Check sheet for the drawn part. Datum: minimum x, y, z corner. Units: mm. A direction names the side the tool comes from. Coordinates: 2 decimals unless noted, no trailing zeros. Order: outer loops, then holes, each group sorted by start corner. A loop starts at its lowest first (then second) coordinate and runs counter-clockwise, first axis right, second up. Notation, with made-up numbers: M 49.25,-23.75 L 75.25,-23.75 A26 cw 75.25,-3.75 Z; hole C 31.25,-30 d1. An arc over 180 degrees is marked long. Return JSON: item names as keys, results as strings. Group by question number.
Q1. Section check B-B, the plane z = 14.5. Enter the section's corners in (x, y) (1 decimal).
Q2. Mould release check, pull along Z, two halves, no side actions. Record for the marked faces 1, 2, 3 and 4: pulls with the +Z half, pulls with the -Z half, needs draft (parallel to the pull), parting line crosses it, or undercut.
Q3. Go/stop test with flat-tipped pins: pin 1 Ø14 at (x, z) = (15, 13.5) entering from -Y; pin 2 Ø0.9 at (x, y) = (11.5, 1) entering from +Z; pin 3 Ø5.5 at (x, z) = (12.5, 12.5) entering from +Y. Record where each tip stops, or that it passes through.
Q4. Thickness scan on probe 1 along X at (y, z) = (4.05, 12.5); probe 2 along Z at (x, y) = (12.75, 2.85); probe 3 along Y at (x, z) = (14.5, 18.75). Record the ranges inside material, lowest first.
Q5. Section check D-D, the plane z = 6.5. Enter the section's corners in (x, y) (1 decimal).
Q6. Section check A-A, the plane x = 12.5. Enter the section's corners in (y, z).
Q7. Section check C-C, the plane y = 2.7. Enter the section's corners in (x, z) (1 decimal), then the cut area to 3 significant figures.
Q8. Access from +Z, -Z, +X, -X, +Y, -Y to the whole of each face (thin tool, end or side, straight path). Record for the marked faces 5 and 6.
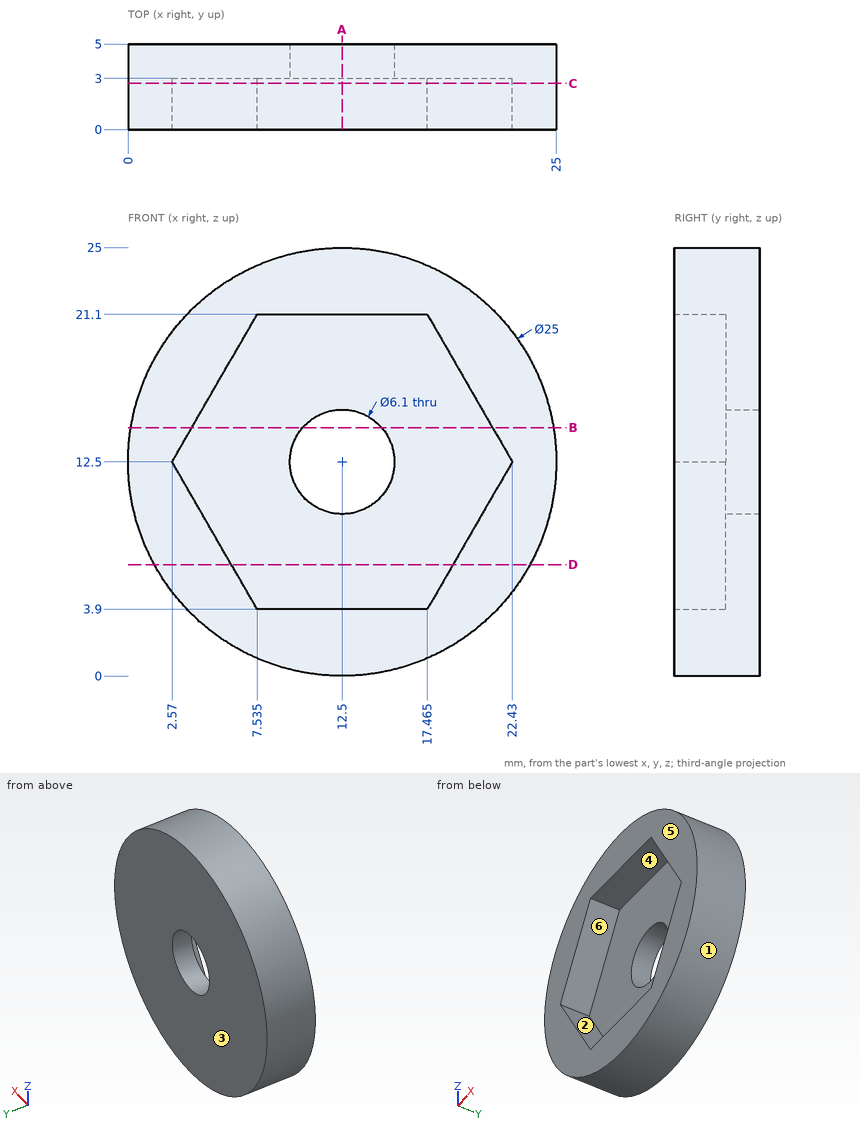
Numbers:
{
 "1": {"outline": "M 0.2,0 L 3.7,0 L 3.7,3 L 10.2,3 L 10.2,5 L 0.2,5 Z; M 14.8,3 L 21.3,3 L 21.3,0 L 24.8,0 L 24.8,5 L 14.8,5 Z"},
 "2": {"face 1": "parting line crosses it", "face 2": "undercut", "face 3": "needs draft", "face 4": "undercut"},
 "3": {"pin 1": "stops at y = 0", "pin 2": "stops at z = 24.99", "pin 3": "passes through"},
 "4": {"probe 1": "x = 0 to 9.45, 15.55 to 25", "probe 2": "z = 0 to 3.9, 21.1 to 25", "probe 3": "y = 3 to 5"},
 "5": {"outline": "M 1.5,0 L 6,0 L 6,3 L 19,3 L 19,0 L 23.5,0 L 23.5,5 L 1.5,5 Z"},
 "6": {"outline": "M 0,0 L 5,0 L 5,9.45 L 3,9.45 L 3,3.9 L 0,3.9 Z; M 0,21.1 L 3,21.1 L 3,15.55 L 5,15.55 L 5,25 L 0,25 Z"},
 "7": {"outline": "C 12.5,12.5 d25; hole M 2.6,12.5 L 7.5,3.9 L 17.5,3.9 L 22.4,12.5 L 17.5,21.1 L 7.5,21.1 Z", "area": "235 mm2"},
 "8": {"face 5": "+Z, -Z, +X, -X, -Y", "face 6": "-Y"}
}
